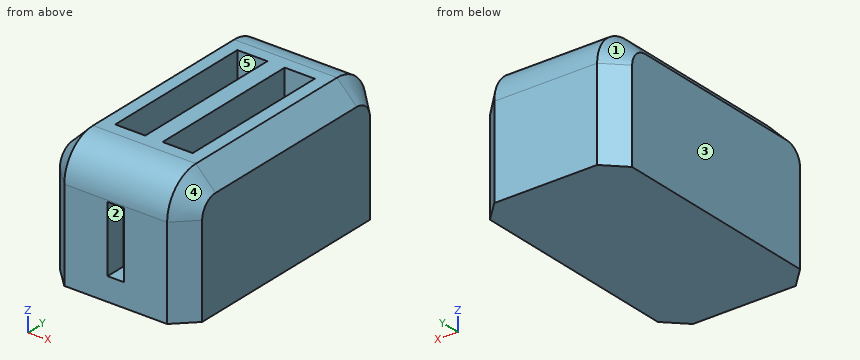
from build123d import *

# Parameters (mm, degrees)
F0_W     = 73.3732283115
F0_H     = 131.3513368368
F1_DEPTH = 66.04
F2_R     = 19.0095175901
F3_SIZE  = 10.16
F4_W     = 15.4954213649
F4_H     = 80.7549729943
F5_DEPTH = 59.436
F7_START = -19.812
F6_W     = 8.3436891437
F6_H     = 37.5465899706
F7_DEPTH = 34.29


with BuildPart() as f1:
    # F0 (on Top) → F1 (new body)
    with BuildSketch(Plane.XY):
        Rectangle(F0_W, F0_H)
    extrude(amount=F1_DEPTH)

    # F2
    f2_edges = [f1.edges().sort_by_distance(p)[0] for p in [
        (0, 65.675668, 66.04),
        (0, -65.675668, 66.04),
    ]]
    fillet(f2_edges, radius=F2_R)

    # F3
    f3_edges = [f1.edges().sort_by_distance(p)[0] for p in [
        (-36.686614, 0, 66.04),
        (-36.686614, 60.10791, 60.472241),
        (-36.686614, 65.675668, 23.515241),
        (-36.686614, -60.10791, 60.472241),
        (-36.686614, -65.675668, 23.515241),
        (36.686614, 0, 66.04),
        (36.686614, 60.10791, 60.472241),
        (36.686614, 65.675668, 23.515241),
        (36.686614, -60.10791, 60.472241),
        (36.686614, -65.675668, 23.515241),
    ]]
    chamfer(f3_edges, length=F3_SIZE)

    # F4 (on face) → F5 (cut)
    with BuildSketch(Plane.XY.offset(66.04)):
        with Locations((12.2175393626, 0)):
            Rectangle(F4_W, F4_H)
        with Locations((-12.2175393626, 0)):
            Rectangle(F4_W, F4_H)
    extrude(amount=-F5_DEPTH, mode=Mode.SUBTRACT)

    # F6 (on face) → F7 (cut)
    with BuildSketch(Plane.XY.offset(66.04).offset(F7_START)):
        with Locations((0, -74.0502253175)):
            Rectangle(F6_W, F6_H)
    extrude(amount=-F7_DEPTH, mode=Mode.SUBTRACT)


solid = f1.part
Can you work these out from the model? Positions are in its coordinate system, mm. Face numbers are marked on the shaded views. A direction names the side the tool comes from. Give positions to 0.01 mm unless a question says otherwise; leave off trailing zeros. Loops run counter-clockwise (first coordinate to the right, second up) from the corner with the lowest first, then second, coordinate; pieces in that order, holes last. Notation, with made-up numbers: (13, 73) -> (27, 73) arc R14 ccw to (27, 80) -> close; hole circle Ø9 at (43, 41.5). An arc over 180 degrees is marked (long way). Use one line per item in the form item = value.
1) If we section it at C-C (y = 45): Please give me the cut outline in (x, z), plus the area to 3 significant figures.
Answers:
outline = (-36.69, 0) -> (36.69, 0) -> (36.69, 55.88) -> (26.53, 66.04) -> (-26.53, 66.04) -> (-36.69, 55.88) -> close
area = 4,740 mm²
2) For the marked faces 4 and 5, which set-ups out of +Z, -Z, +X, -X, +Y, -Y let a thin tool reach every point of the face, with its end or its side?
Answers:
face_4 = +Z, +X, -Y
face_5 = +Z
3) We'd pull the mould along Z, two halves only. Please class the marked faces 1, 2 and 3: released by +Z, released by -Z, zero draft, split by the parting line, or undercut.
Answers:
face_1 = released by +Z
face_2 = undercut
face_3 = zero draft
4) If we section it at B-B (x = -7): Please give me the cut outline in (y, z), plus the area to 3 significant figures.
Answers:
outline = (-65.68, 0) -> (65.68, 0) -> (65.68, 47.03) arc R19.01 ccw to (46.67, 66.04) -> (40.38, 66.04) -> (40.38, 6.6) -> (-40.38, 6.6) -> (-40.38, 66.04) -> (-46.67, 66.04) arc R19.01 ccw to (-65.68, 47.03) -> close
area = 3,720 mm²
5) Will these pins go through, and if not, where does the flat tip stop? pin 1 (9 mm diameter, centred on x = -1, y = -59.5, fed in from +Z); pin 2 (5 mm diameter, centred on y = -62, z = 37.5, fed in from -X); pin 3 (7.5 mm diameter, centred on x = 11, y = -14.5, fed in from +Z).
Answers:
pin_1 = 64.12
pin_2 = -32.7
pin_3 = 6.6
6) If we section it at D-D (z = 17): Please give me the cut outline in (x, y), plus the area to 3 significant figures.
Answers:
outline = (-36.69, -55.52) -> (-26.53, -65.68) -> (-4.17, -65.68) -> (-4.17, -55.28) -> (4.17, -55.28) -> (4.17, -65.68) -> (26.53, -65.68) -> (36.69, -55.52) -> (36.69, 55.52) -> (26.53, 65.68) -> (-26.53, 65.68) -> (-36.69, 55.52) -> close; hole (-19.97, -40.38) -> (-4.47, -40.38) -> (-4.47, 40.38) -> (-19.97, 40.38) -> close; hole (4.47, -40.38) -> (19.97, -40.38) -> (19.97, 40.38) -> (4.47, 40.38) -> close
area = 6,840 mm²
7) I need wall thicknesses on line 1 along X through (y, z) = (-27, 24.5); line 2 along Y through (x, z) = (-18, 18); line 3 along Z through (x, y) = (-16, -21). Which ranges of each line are inside material? Lowest first, please.
Answers:
line_1 = -36.69 to -19.97, -4.47 to 4.47, 19.97 to 36.69
line_2 = -65.68 to -40.38, 40.38 to 65.68
line_3 = 0 to 6.6
8) If we section it at A-A (z = 9): Please give me the cut outline in (x, y).
Answers:
outline = (-36.69, -55.52) -> (-26.53, -65.68) -> (26.53, -65.68) -> (36.69, -55.52) -> (36.69, 55.52) -> (26.53, 65.68) -> (-26.53, 65.68) -> (-36.69, 55.52) -> close; hole (-19.97, -40.38) -> (-4.47, -40.38) -> (-4.47, 40.38) -> (-19.97, 40.38) -> close; hole (4.47, -40.38) -> (19.97, -40.38) -> (19.97, 40.38) -> (4.47, 40.38) -> close
